```python
from build123d import *

# Parameters (mm, degrees)
F0_W     = 101.6
F0_H     = 6.35
F1_DEPTH = 6.35


with BuildPart() as f1:
    # F0 (on Top) → F1 (new body)
    with BuildSketch(Plane.XY):
        Polygon((-63.5, 63.5), (-76.2, 63.5), (-76.2, 57.15), (-76.2, 50.8), (-76.2, 44.45), (-76.2, 38.1), (-76.2, 31.75), (-76.2, 25.4), (-76.2, 19.05), (-69.85, 19.05), (-69.85, 12.7), (-69.85, 6.35), (-69.85, 0), (-69.85, -6.35), (-69.85, -12.7), (-76.2, -12.7), (-76.2, -19.05), (-76.2, -25.4), (-76.2, -31.75), (-76.2, -38.1), (-76.2, -44.45), (-76.2, -50.8), (-76.2, -57.15), (-69.85, -57.15), (-63.5, -57.15), (-57.15, -57.15), (-50.8, -57.15), (-44.45, -57.15), (-38.1, -57.15), (-31.75, -57.15), (-25.4, -57.15), (-19.05, -57.15), (-19.05, -63.5), (-12.7, -63.5), (-6.35, -63.5), (0, -63.5), (6.35, -63.5), (12.7, -63.5), (12.7, -57.15), (19.05, -57.15), (25.4, -57.15), (31.75, -57.15), (38.1, -57.15), (44.45, -57.15), (50.8, -57.15), (57.15, -57.15), (63.5, -57.15), (69.85, -57.15), (69.85, -50.8), (69.85, -44.45), (69.85, -38.1), (69.85, -31.75), (69.85, -25.4), (69.85, -19.05), (69.85, -12.7), (76.2, -12.7), (76.2, -6.35), (76.2, 0), (76.2, 6.35), (76.2, 12.7), (76.2, 19.05), (69.85, 19.05), (69.85, 25.4), (69.85, 31.75), (69.85, 38.1), (69.85, 44.45), (69.85, 50.8), (69.85, 63.5), (63.5, 63.5), (57.15, 63.5), (50.8, 63.5), (44.45, 63.5), (38.1, 63.5), (31.75, 63.5), (25.4, 63.5), (19.05, 63.5), (12.7, 63.5), (12.7, 57.15), (6.35, 57.15), (0, 57.15), (-6.35, 57.15), (-12.7, 57.15), (-19.05, 57.15), (-19.05, 63.5), (-25.4, 63.5), (-31.75, 63.5), (-38.1, 63.5), (-44.45, 63.5), (-50.8, 63.5), (-57.15, 63.5), align=None)
        Rectangle(F0_W, F0_H, mode=Mode.SUBTRACT)
    extrude(amount=F1_DEPTH)


solid = f1.part
```
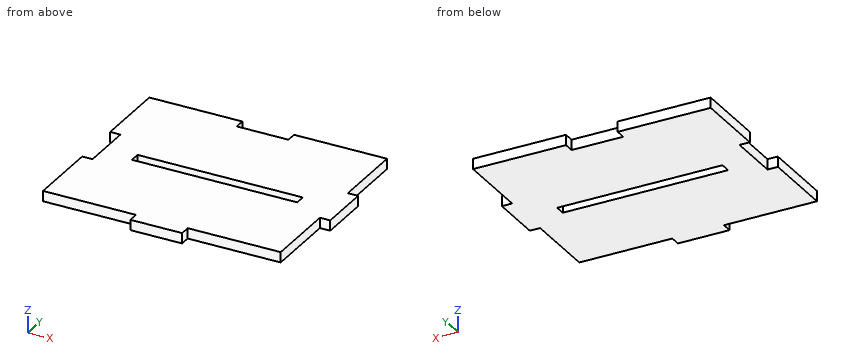
CAD build for the part. Positions are in the model's coordinates, mm. Coordinates: 2 decimals unless noted, no trailing zeros. Write each loop counter-clockwise with the first axis right and the second up, starting at its lowest first coordinate (ties: lowest second). Pieces come first, ordered by that corner, then holes. Notation, with made-up numbers: (-37.75, 89.25) -> (-27.75, 89.25) arc R25 cw to (-27.75, 106.25) -> close; hole circle Ø2 at (40.25, 57.5). An arc over 180 degrees is marked (long way). Return JSON: item names as keys, results as strings. Group by question number.
Q1. Cut at A-A, the plane z = 5. Give the cut face in (x, y) (3 decimals).
Q2. Flat gauge pins, fed straight in: pin 1 (1 mm diameter, centred on x = 50, z = 4.5, fed in from -Y); pin 2 (1.9 mm diameter, centred on x = 74, z = 3.5, fed in from +Y); pin 3 (3 mm diameter, centred on y = 0, z = 3, fed in from -X). Where does each tip first touch, or does it go through?
Q3. Drill centre lines: line 1 (Y direction, x = 34, z = 2) (3 decimals); line 2 (Y direction, x = 12, z = 2) (3 decimals); line 3 (X direction, y = -38.5, z = 2.25). Where is each one in solid material? Low to high.
Q4. Cut at B-B, the plane x = 7. Give the cut face in (y, z) (3 decimals), then the cut area to 3 significant figures.
Q5. Cut at D-D, the plane y = -8. Give the cut face in (x, z), then the cut area to 3 significant figures.
Q6. Cut at C-C, the plane y = 39. Give the cut face in (x, z), then the cut area to 3 significant figures.
Returned:
{
 "1": {"outline": "(-76.2, -57.15) -> (-19.05, -57.15) -> (-19.05, -63.5) -> (12.7, -63.5) -> (12.7, -57.15) -> (69.85, -57.15) -> (69.85, -12.7) -> (76.2, -12.7) -> (76.2, 19.05) -> (69.85, 19.05) -> (69.85, 63.5) -> (12.7, 63.5) -> (12.7, 57.15) -> (-19.05, 57.15) -> (-19.05, 63.5) -> (-76.2, 63.5) -> (-76.2, 19.05) -> (-69.85, 19.05) -> (-69.85, -12.7) -> (-76.2, -12.7) -> close; hole (-50.8, -3.175) -> (50.8, -3.175) -> (50.8, 3.175) -> (-50.8, 3.175) -> close"},
 "2": {"pin 1": "stops at y = -57.15", "pin 2": "stops at y = 19.05", "pin 3": "stops at x = -69.85"},
 "3": {"line 1": "y = -57.15 to -3.175, 3.175 to 63.5", "line 2": "y = -63.5 to -3.175, 3.175 to 57.15", "line 3": "x = -76.2 to 69.85"},
 "4": {"outline": "(-63.5, 0) -> (-3.175, 0) -> (-3.175, 6.35) -> (-63.5, 6.35) -> close; (3.175, 0) -> (57.15, 0) -> (57.15, 6.35) -> (3.175, 6.35) -> close", "area": "726 mm2"},
 "5": {"outline": "(-69.85, 0) -> (76.2, 0) -> (76.2, 6.35) -> (-69.85, 6.35) -> close", "area": "927 mm2"},
 "6": {"outline": "(-76.2, 0) -> (69.85, 0) -> (69.85, 6.35) -> (-76.2, 6.35) -> close", "area": "927 mm2"}
}
